```python
from build123d import *

# Parameters (mm, degrees)
SKIZZE1_W                       = 70
SKIZZE1_H                       = 50
AUFSATZ_LINEAR_AUSTRAGEN1_DEPTH = 10
SKIZZE2_W                       = 50.5
SKIZZE2_H                       = 40.5
SCHNITT_LINEAR_AUSTRAGEN1_DEPTH = 5
FASE2_SIZE                      = 5


with BuildPart() as part:
    # Skizze1 → Aufsatz-Linear austragen1 (new body)
    with BuildSketch(Plane.XY):
        Rectangle(SKIZZE1_W, SKIZZE1_H)
    extrude(amount=AUFSATZ_LINEAR_AUSTRAGEN1_DEPTH)

    # Skizze2 → Schnitt-Linear austragen1 (cut)
    with BuildSketch(Plane.XY.offset(10)):
        Rectangle(SKIZZE2_W, SKIZZE2_H)
    extrude(amount=-SCHNITT_LINEAR_AUSTRAGEN1_DEPTH, mode=Mode.SUBTRACT)

    # Fase2
    fase2_edges = [part.edges().sort_by_distance(p)[0] for p in [
        (35, 0, 10),
        (-35, 0, 10),
    ]]
    chamfer(fase2_edges, length=FASE2_SIZE)


solid = part.part
```
Geometry: final body of the model. Coordinates: model frame, mm. A direction names the side the tool comes from. Round coordinates to 2 decimals unless told otherwise and drop trailing zeros. Order: outer loops, then holes, each group sorted by start corner. A loop starts at its lowest first (then second) coordinate and runs counter-clockwise, first axis right, second up. Notation, with made-up numbers: (-30.5, -11.75) - (-13.5, -11.75) arc R28 ccw to (-13.5, 27.25) - close; hole circle Ø7 at (69, -25.75). An arc over 180 degrees is marked (long way). Use CSV: the item, a comma, the result in double quotes. Start each with the question number.
Q1. Mould query, pull axis X, two halves, no side actions, for faces 3 (the face through (0, -22, 10)), 4 (the face through (25.25, 0, 8)), 5 (the face through (35, 0, 2)), 6 (the face through (0, 20.25, 8)). Classes: +X half, -X half, draft (parallel to the pull), parting line (faces both ways), or undercut.
Q2. Material intervals for line 1 along Y through (x, z) = (8.5, 6.5); line 2 along Z through (x, y) = (-24.5, 11); line 3 along X through (y, z) = (4, 9), sorted ascending. Write a range as from..to.
Q3. Section query C-C (y = -7). Return loops of the section in (x, z).
Q4. Section query B-B (x = 21). Return loops of the section in (y, z), and give its area (4 significant figures).
Q5. Access query for faces 1 (the face through (33, 0, 7)), 2 (the face through (0, 0, 5)). Directions: +Z, -Z, +X, -X, +Y, -Y. A direction counts if a zero-diameter tool reaches every point of the face in a straight line with its end or side. Return the directions, or none.
Q6. Section query A-A (z = 7.5). Return loops of the section in (x, y).
Q7. First-contact query: pin 1 (1 mm diameter, centred on x = 13, y = -2, fed in from +Z); pin 2 (1.5 mm diameter, centred on y = 15, z = 7.5, fed in from -X); pin 3 (5.5 mm diameter, centred on y = 8.5, z = 7.5, fed in from +X); pin 4 (2.5 mm diameter, centred on y = -4, z = 7, fed in from -X). Flat tips, straight axial feed; report the tip coordinate or a pass-through.
Result set:
1,face 3,"draft"
1,face 4,"undercut"
1,face 5,"+X half"
1,face 6,"undercut"
2,line 1,"y = -25..-20.25, 20.25..25"
2,line 2,"z = 0..5"
2,line 3,"x = -31..-25.25, 25.25..31"
3,outline,"(-35, 0) - (35, 0) - (35, 5) - (30, 10) - (25.25, 10) - (25.25, 5) - (-25.25, 5) - (-25.25, 10) - (-30, 10) - (-35, 5) - close"
4,outline,"(-25, 0) - (25, 0) - (25, 10) - (20.25, 10) - (20.25, 5) - (-20.25, 5) - (-20.25, 10) - (-25, 10) - close"
4,area,"297.5 mm2"
5,face 1,"+Z, +X, +Y, -Y"
5,face 2,"+Z"
6,outline,"(-32.5, -25) - (32.5, -25) - (32.5, 25) - (-32.5, 25) - close; hole (-25.25, -20.25) - (25.25, -20.25) - (25.25, 20.25) - (-25.25, 20.25) - close"
7,pin 1,"stops at z = 5"
7,pin 2,"stops at x = -33.25"
7,pin 3,"stops at x = 35"
7,pin 4,"stops at x = -34.25"
